Geometry: final body of the model. Coordinates: model frame, mm. A direction names the side the tool comes from. Round coordinates to 2 decimals unless told otherwise and drop trailing zeros. Order: outer loops, then holes, each group sorted by start corner. A loop starts at its lowest first (then second) coordinate and runs counter-clockwise, first axis right, second up. Notation, with made-up numbers: (0.25, 83.5) -> (31.25, 83.5) arc R14 ccw to (31.25, 98.5) -> close; hole circle Ø6 at (-23, 13.25). An arc over 180 degrees is marked (long way). Put each result on its own line as item: value.
```python
from build123d import *

# Parameters (mm, degrees)
F0_W     = 15.24
F0_H     = 12.7
F1_DEPTH = 6.35


# Not quite as in the source:
# - a feature names something its author has since deleted; it is built from what else it names


with BuildPart() as f1:
    # F0 (on Front) → F1 (new body, symmetric)
    with BuildSketch(Plane.XZ):
        Polygon((-11.5497628391, 12.7), (-17.8997628391, 0), (10.0402371609, 0), (10.0402371609, 12.7), align=None)
        with BuildLine():
            Line((10.0402371609, 12.7), (10.0402371609, 0))
            ThreePointArc((10.0402371609, 0), (29.0902371609, 19.05), (10.0402371609, 38.1))
            Line((10.0402371609, 38.1), (10.0402371609, 25.4))
            ThreePointArc((10.0402371609, 25.4), (16.3902371609, 19.05), (10.0402371609, 12.7))
        make_face()
        with Locations((2.4202371609, 31.75)):
            Rectangle(F0_W, F0_H)
        with BuildLine():
            Line((-5.1997628391, 25.4), (-5.1997628391, 38.1))
            Line((-5.1997628391, 38.1), (-17.8997628391, 38.1))
            ThreePointArc((-17.8997628391, 38.1), (-14.1800189601, 29.1197438789), (-5.1997628391, 25.4))
        make_face()
    extrude(amount=F1_DEPTH, both=True)


solid = f1.part
```
1. Set-up query: faces 1 (the face through (2, 0, 25.4)), 2 (the face through (-4, 0, 0)). Return all of +Z, -Z, +X, -X, +Y, -Y with unobstructed straight access to the full face (end or side cutting, diameter ignored); none if empty.
Ans:
face 1: -X, +Y, -Y
face 2: -Z, +X, -X, +Y, -Y
2. Draft query along Z for faces 3 (the face through (-4, 0, 38.1)), 4 (the face through (5, 6.35, 28)), 5 (the face through (-14.28, -0.09, 29.22)). Return one class per face: +Z half, -Z half, draft (parallel to the pull), parting line (faces both ways), or undercut.
Ans:
face 3: +Z half
face 4: draft
face 5: undercut
3. Cut plane B-B on y = -3. Return loops of the section in (x, z).
Ans:
outline: (-17.9, 0) -> (10.04, 0) arc R19.05 ccw to (10.04, 38.1) -> (-17.9, 38.1) arc R12.7 ccw to (-5.2, 25.4) -> (10.04, 25.4) arc R6.35 cw to (10.04, 12.7) -> (-11.55, 12.7) -> close
4. Contact query for a flat-ended pin moving along its axis: P1, Ø4, axis at y = 1.5, z = 13.5, coming from the -X side. Output: stop coordinate, or through.
Ans:
P1: x = -12.15
5. Cut plane C-C on z = 19.05. Return loops of the section in (x, y).
Ans:
outline: (16.39, -6.35) -> (29.09, -6.35) -> (29.09, 6.35) -> (16.39, 6.35) -> close
6. Material intervals for probe 1 along Z at (x, y) = (0, -4); probe 2 along Z at (x, y) = (-6.5, -0.5); probe 3 along X at (y, z) = (-0.75, 22.5), sorted ascending.
Ans:
probe 1: 0 to 12.7, 25.4 to 38.1
probe 2: 0 to 12.7, 25.47 to 38.1
probe 3: 15.37 to 28.78
7. Cut plane A-A on x = 9. Return loops of the section in (y, z).
Ans:
outline: (-6.35, 0) -> (6.35, 0) -> (6.35, 12.7) -> (-6.35, 12.7) -> close; (-6.35, 25.4) -> (6.35, 25.4) -> (6.35, 38.1) -> (-6.35, 38.1) -> close
8. Cut plane D-D on x = 21. Return loops of the section in (y, z).
Ans:
outline: (-6.35, 3.47) -> (6.35, 3.47) -> (6.35, 34.63) -> (-6.35, 34.63) -> close
